Check sheet for the modelled part. Datum: model origin and axes. Units: mm. Face numbers are marked on the shaded views. A direction names the side the tool comes from. Give positions to 0.01 mm unless a question says otherwise; leave off trailing zeros. Write each loop counter-clockwise with the first axis right and the second up, starting at its lowest first coordinate (ties: lowest second). Pieces come first, ordered by that corner, then holes. Notation, with made-up numbers: M 37.25,72.25 L 69.25,72.25 A22 ccw 69.25,93.25 Z; hole C 31.5,-11 d2. An arc over 180 degrees is marked long. Write item = value, one per line. Start each with the question number.
1) Access from +Z, -Z, +X, -X, +Y, -Y to the whole of each face (thin tool, end or side, straight path). Record for the marked faces 4, 5 and 6.
2) Cross-section at A-A, the plane y = 0.75. Record the cut outline in (x, z).
3) Cross-section at C-C, the plane x = -17.5. Record the cut outline in (y, z), plus the area to 3 significant figures.
4) Go/stop test with flat-tipped pins: pin 1 (8 mm diameter, centred on x = -31.5, z = -3.5, fed in from -Y); pin 2 (1.5 mm diameter, centred on y = -12.5, z = -2, fed in from -X); pin 3 (2 mm diameter, centred on x = -30.5, y = -5.5, fed in from -Z). Record where each tip stops, or that it passes through.
5) Mould release check, pull along Y, two halves, no side actions. Record for the marked faces 1, 2 and 3: released by +Y, released by -Y, zero draft, split by the parting line, or undercut.
6) Scan lines: line 1 along Y through (x, z) = (-16, 3.25); line 2 along X through (y, z) = (-11.25, -5.5); line 3 along X through (y, z) = (1.25, -1.5). Record each from-to range of solid material in increasing order. Write a range as [from, to].
```python
from build123d import *

# Parameters (mm, degrees)
F0_W     = 15.5
F0_H     = 15.5
F1_DEPTH = 7.5
F2_R     = 9.99999


# Not quite as in the source:
# - a fillet or chamfer is up to 0.001 mm smaller than in the source, because OpenCascade refuses the exact size
# - a feature names something its author has since deleted; it is built from what else it names


with BuildPart() as f1:
    # F0 (on Top) → F1 (new body, symmetric)
    with BuildSketch(Plane.XY):
        Polygon((-25.621605996, -0.5219928448), (-25.621605996, -7.0219928448), (-25.621605996, -13.5219928448), (-6.621605996, -13.5219928448), (-6.621605996, -8.299067306), (-6.621605996, 4.9780071552), (-35.621605996, 4.9780071552), (-35.621605996, 2.9780071552), (-25.621605996, 2.9780071552), (-25.621605996, 1.4780071552), (-35.621605996, 1.4780071552), (-35.621605996, -0.5219928448), align=None)
        with Locations((-15.871605996, -4.2719928448)):
            Rectangle(F0_W, F0_H, mode=Mode.SUBTRACT)
    extrude(amount=F1_DEPTH, both=True)

    # F2 (radius 10 in the source; OpenCascade refuses exactly that, so slightly less here)
    f2_edges = [f1.edges().sort_by_distance(p)[0] for p in [
        (-25.621606, -0.521993, 0),
    ]]
    fillet(f2_edges, radius=F2_R)


solid = f1.part
```
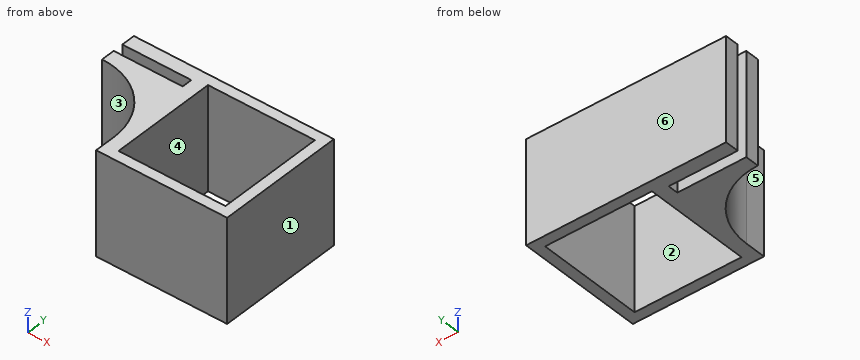
Reply:
q1.face_4 = +Z, -Z
q1.face_5 = +Z, -Z, -X, -Y
q1.face_6 = +Z, -Z, +X, -X, +Y
q2.outline = M -35.62,-7.5 L -23.62,-7.5 L -23.62,7.5 L -35.62,7.5 Z; M -8.12,-7.5 L -6.62,-7.5 L -6.62,7.5 L -8.12,7.5 Z
q3.outline = M -13.52,-7.5 L -12.02,-7.5 L -12.02,7.5 L -13.52,7.5 Z; M 3.48,-7.5 L 4.98,-7.5 L 4.98,7.5 L 3.48,7.5 Z
q3.area = 45.0 mm2
q4.pin_1 = -4.69
q4.pin_2 = -25.62
q4.pin_3 = through
q5.face_1 = zero draft
q5.face_2 = undercut
q5.face_3 = released by -Y
q6.line_1 = [-13.52, -12.02], [3.48, 4.98]
q6.line_2 = [-25.62, -23.62], [-8.12, -6.62]
q6.line_3 = [-35.62, -23.62], [-8.12, -6.62]
